Can you work these out from the drawing? Everything is in mm from the part's minimum corner. A direction names the side the tool comes from. Give positions to 0.01 mm unless a question says otherwise; leave off trailing zeros. Order: outer loops, then holes, each group sorted by start corner. A loop starts at its lowest first (then second) coordinate and runs counter-clockwise, first axis right, second up. Notation, with made-up numbers: (24.5, 74) - (32.5, 74) arc R19 cw to (32.5, 82) - close; hole circle Ø11 at (20, 40.5). An arc over 180 degrees is marked (long way). Answer as a JSON object with one key per item and string values.
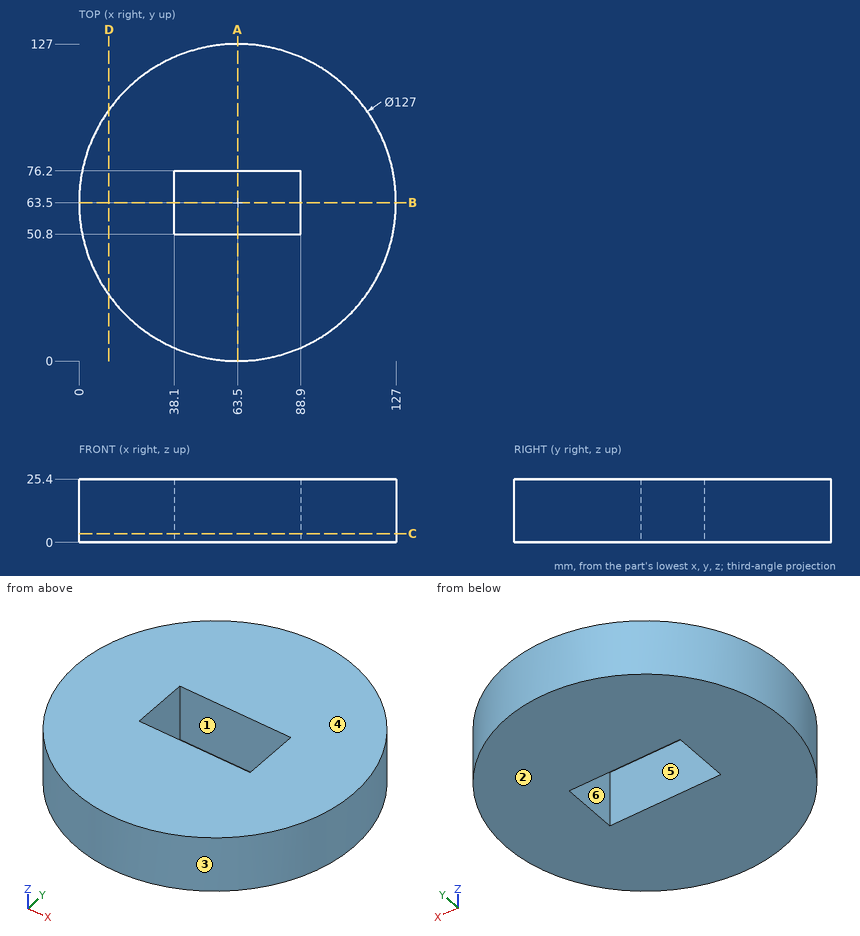
Q1. If we section it at A-A, the plane x = 63.5: Please give me the cut outline in (y, z), then the cut area to 3 significant figures.
Recorded:
{"outline": "(0, 0) - (50.8, 0) - (50.8, 25.4) - (0, 25.4) - close; (76.2, 0) - (127, 0) - (127, 25.4) - (76.2, 25.4) - close", "area": "2,580 mm^2"}
Q2. If we section it at D-D, the plane x = 12: Please give me the cut outline in (y, z).
Recorded:
{"outline": "(26.35, 0) - (100.65, 0) - (100.65, 25.4) - (26.35, 25.4) - close"}
Q3. Which directions (+Z, -Z, +X, -X, +Y, -Y) give clear straight access to the entire face, cutting with the end or side of a thin tool? Please do the marked faces 1 and 2.
Recorded:
{"face 1": "+Z, -Z", "face 2": "-Z, +X, -X, +Y, -Y"}
Q4. We'd pull the mould along Y, two halves only. Please class the marked faces 3, 4, 5 and 6: released by +Y, released by -Y, zero draft, split by the parting line, or undercut.
Recorded:
{"face 3": "split by the parting line", "face 4": "zero draft", "face 5": "undercut", "face 6": "undercut"}
Q5. I need wall thicknesses on L1, parallel to X at y = 64, z = 7.5; L2, parallel to Y at x = 86.5, z = 13.75; L3, parallel to Y at x = 85, z = 21.5. Which ranges of each line are inside material? Lowest first, please.
Recorded:
{"L1": "x = 0 to 38.1, 88.9 to 127", "L2": "y = 4.31 to 50.8, 76.2 to 122.69", "L3": "y = 3.75 to 50.8, 76.2 to 123.25"}
Q6. If we section it at C-C, the plane z = 3.5: Please give me the cut outline in (x, y).
Recorded:
{"outline": "circle Ø127 at (63.5, 63.5); hole (38.1, 50.8) - (88.9, 50.8) - (88.9, 76.2) - (38.1, 76.2) - close"}
Q7. If we section it at B-B, the plane y = 63.5: Please give me the cut outline in (x, z).
Recorded:
{"outline": "(0, 0) - (38.1, 0) - (38.1, 25.4) - (0, 25.4) - close; (88.9, 0) - (127, 0) - (127, 25.4) - (88.9, 25.4) - close"}
Q8. I'm going to push flat-ended pins straight in: pin 1 Ø1 at (y, z) = (84, 9) entering from +X; pin 2 Ø5 at (x, z) = (57.5, 4) entering from -Y; pin 3 Ø1.5 at (x, z) = (89, 7.5) entering from +Y. Where does each tip first touch, or does it pass through?
Recorded:
{"pin 1": "stops at x = 123.77", "pin 2": "stops at y = 0.1", "pin 3": "stops at y = 121.98"}
